from build123d import *

# Parameters (mm, degrees)
SKETCH1_W           = 204.3
SKETCH1_H           = 173.7
BOSS_EXTRUDE2_DEPTH = 10
SKETCH4_W           = 204.3
SKETCH4_H           = 15
BOSS_EXTRUDE4_DEPTH = 68.9
SKETCH6_W           = 204.3
SKETCH6_H           = 5
CUT_EXTRUDE1_DEPTH  = 26
SKETCH5_W           = 204.3
SKETCH5_H           = 15
BOSS_EXTRUDE6_DEPTH = 7.3
FILLET1_R           = 20
SKETCH7_W           = 143.7
SKETCH7_H           = 7.3
BOSS_EXTRUDE7_DEPTH = 204.3
SKETCH9_W           = 158.7
SKETCH9_H           = 7.9
BOSS_EXTRUDE9_DEPTH = 1.3


with BuildPart() as part:
    # Sketch1 → Boss-Extrude2 (new body)
    with BuildSketch(Plane(origin=(0, 0, 0), x_dir=(1, 0, 0), z_dir=(0, 1, 0))):
        with Locations((272.329166667, 26.170833333)):
            Rectangle(SKETCH1_W, SKETCH1_H)
    extrude(amount=BOSS_EXTRUDE2_DEPTH)

    # Sketch4 → Boss-Extrude4 (add)
    with BuildSketch(Plane(origin=(0, 0, 0), x_dir=(-1, 0, 0), z_dir=(0, -1, 0))):
        with Locations((-272.329166667, 105.520833333)):
            Rectangle(SKETCH4_W, SKETCH4_H)
    extrude(amount=BOSS_EXTRUDE4_DEPTH)

    # Sketch6 → Cut-Extrude1 (cut)
    with BuildSketch(Plane.XY.offset(-98.020833333)):
        with Locations((272.329166667, -66.4)):
            Rectangle(SKETCH6_W, SKETCH6_H)
    extrude(amount=-CUT_EXTRUDE1_DEPTH, mode=Mode.SUBTRACT)

    # Sketch5 → Boss-Extrude6 (add)
    with BuildSketch(Plane.XZ):
        with Locations((272.329166667, 53.179166667)):
            Rectangle(SKETCH5_W, SKETCH5_H)
    extrude(amount=BOSS_EXTRUDE6_DEPTH)

    # Fillet1
    fillet1_edges = [part.edges().sort_by_distance(p)[0] for p in [
        (272.329166667, 10, -113.020833333),
    ]]
    fillet(fillet1_edges, radius=FILLET1_R)

    # Sketch7 → Boss-Extrude7 (add)
    with BuildSketch(Plane(origin=(374.479166667, 0, 0), x_dir=(0, 0, -1), z_dir=(1, 0, 0))):
        with Locations((26.170833333, -3.65)):
            Rectangle(SKETCH7_W, SKETCH7_H)
    extrude(amount=-BOSS_EXTRUDE7_DEPTH)

    # Sketch9 → Boss-Extrude9 (add)
    with BuildSketch(Plane(origin=(374.479166667, 0, 0), x_dir=(0, 0, -1), z_dir=(1, 0, 0))):
        with Locations((18.670833333, -16.85)):
            Rectangle(SKETCH9_W, SKETCH9_H)
    extrude(amount=-BOSS_EXTRUDE9_DEPTH)


solid = part.part
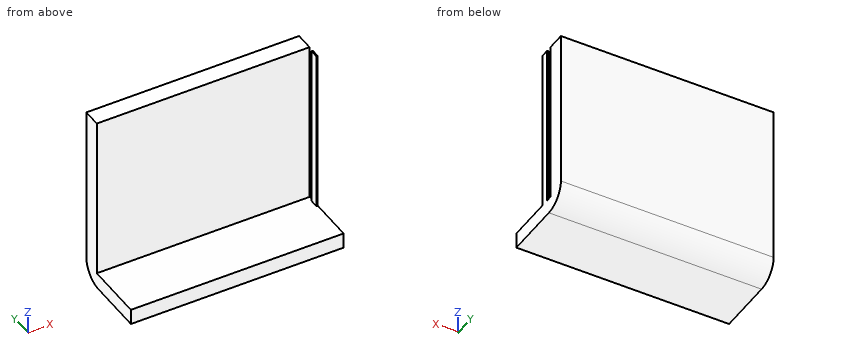
Build history of the part. All positions in model axes, mm. Round coordinates to 2 decimals unless told otherwise and drop trailing zeros. Loops run counter-clockwise (first coordinate to the right, second up) from the corner with the lowest first, then second, coordinate; pieces in that order, holes last. Notation, with made-up numbers: (-25, 82.25) -> (16, 82.25) arc R20 cw to (16, 96.25) -> close; hole circle Ø8 at (-2.75, 19). An arc over 180 degrees is marked (long way). One line per item, written item: value. Start each with the question number.
Q1. Probe line 1 along Y through (x, z) = (188, -12); line 2 along Z through (x, y) = (187, -44.5); line 3 along X through (y, z) = (-20, -51). List the from-to ranges inside material, lowest first.
Q2. Drop flat-ended pins along their axis: pin 1 Ø1.5 at (x, y) = (200.5, -36.5) entering from +Z; pin 2 Ø1 at (x, z) = (374, -25.5) entering from -Y; pin 3 Ø4 at (y, z) = (-16.5, -32.5) entering from -X. Give the stop position or say it passes through.
Q3. Cut at C-C on y = -18. List the corners of the cut face in (x, z), plus the area to 3 significant figures.
Q4. Cut at B-B on x = 285. List the corners of the cut face in (y, z).
Q5. Cut at D-D on y = 1.5. List the corners of the cut face in (x, z), plus the area to 3 significant figures.
Q6. Cut at A-A on z = -74.5. List the corners of the cut face in (x, y).
Computed:
1. line 1: -7.3 to 10
1. line 2: -113.02 to -98.02
1. line 3: 373.18 to 374.48
2. pin 1: z = -98.02
2. pin 2: y = -20.8
2. pin 3: x = 373.18
3. outline: (170.18, -113.02) -> (374.48, -113.02) -> (374.48, 60.68) -> (373.18, 60.68) -> (373.18, -98.02) -> (170.18, -98.02) -> close
3. area: 3,270 mm²
4. outline: (-63.9, -113.02) -> (-10, -113.02) arc R20 ccw to (10, -93.02) -> (10, 60.68) -> (-7.3, 60.68) -> (-7.3, -98.02) -> (-63.9, -98.02) -> close
5. outline: (170.18, -109.38) -> (374.48, -109.38) -> (374.48, 60.68) -> (170.18, 60.68) -> close
5. area: 34,700 mm²
6. outline: (170.18, -7.3) -> (374.48, -7.3) -> (374.48, 10) -> (170.18, 10) -> close; (373.18, -20.8) -> (374.48, -20.8) -> (374.48, -12.9) -> (373.18, -12.9) -> close
